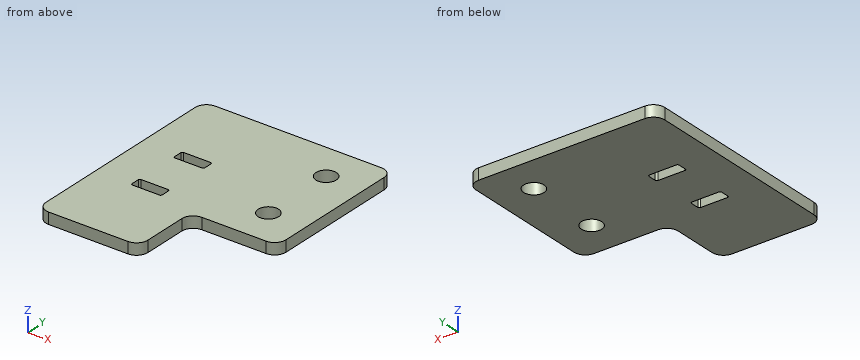
```python
from build123d import *

# Parameters (mm, degrees)
MODEL_R                         = 2.7
AUFSATZ_LINEAR_AUSTRAGEN1_DEPTH = 3


with BuildPart() as part:
    # Model → Aufsatz-Linear austragen1 (new body)
    with BuildSketch(Plane.XY):
        with BuildLine():
            Line((50, 20.75), (50, 54.75))
            ThreePointArc((50, 54.75), (49.121320344, 56.871320344), (47, 57.75))
            Line((47, 57.75), (3, 57.75))
            ThreePointArc((3, 57.75), (0.878679656, 56.871320344), (0, 54.75))
            Line((0, 54.75), (0, 3))
            ThreePointArc((0, 3), (0.878679656, 0.878679656), (3, 0))
            Line((3, 0), (24, 0))
            ThreePointArc((24, 0), (26.121320344, 0.878679656), (27, 3))
            Line((27, 3), (27, 14.75))
            ThreePointArc((27, 14.75), (27.878679656, 16.871320344), (30, 17.75))
            Line((30, 17.75), (47, 17.75))
            ThreePointArc((47, 17.75), (49.121320344, 18.628679656), (50, 20.75))
        make_face()
        with Locations((40, 27.75)):
            Circle(MODEL_R, mode=Mode.SUBTRACT)
        with Locations((40, 47.75)):
            Circle(MODEL_R, mode=Mode.SUBTRACT)
        with BuildLine():
            Line((17.1, 34.75), (9.9, 34.75))
            ThreePointArc((9.9, 34.75), (9.617157288, 34.867157288), (9.5, 35.15))
            Line((9.5, 35.15), (9.5, 37.35))
            ThreePointArc((9.5, 37.35), (9.617157288, 37.632842712), (9.9, 37.75))
            Line((9.9, 37.75), (17.1, 37.75))
            ThreePointArc((17.1, 37.75), (17.382842712, 37.632842712), (17.5, 37.35))
            Line((17.5, 37.35), (17.5, 35.15))
            ThreePointArc((17.5, 35.15), (17.382842712, 34.867157288), (17.1, 34.75))
        make_face(mode=Mode.SUBTRACT)
        with BuildLine():
            Line((17.100000028, 20.000000104), (9.900000028, 20.000000104))
            ThreePointArc((9.900000028, 20.000000104), (9.617157315, 20.117157391), (9.500000028, 20.400000104))
            Line((9.500000028, 20.400000104), (9.500000028, 22.600000104))
            ThreePointArc((9.500000028, 22.600000104), (9.617157315, 22.882842816), (9.900000028, 23.000000104))
            Line((9.900000028, 23.000000104), (17.100000028, 23.000000104))
            ThreePointArc((17.100000028, 23.000000104), (17.38284274, 22.882842816), (17.500000028, 22.600000104))
            Line((17.500000028, 22.600000104), (17.500000028, 20.400000104))
            ThreePointArc((17.500000028, 20.400000104), (17.38284274, 20.117157391), (17.100000028, 20.000000104))
        make_face(mode=Mode.SUBTRACT)
    extrude(amount=AUFSATZ_LINEAR_AUSTRAGEN1_DEPTH)


solid = part.part
```
CAD build for the part. Positions are in the model's coordinates, mm. Round coordinates to 2 decimals unless told otherwise and drop trailing zeros. Order: outer loops, then holes, each group sorted by start corner. A loop starts at its lowest first (then second) coordinate and runs counter-clockwise, first axis right, second up. Notation, with made-up numbers: (16.25, 11.5) - (52.25, 11.5) arc R12 cw to (52.25, 34.5) - close; hole circle Ø6 at (-10, 35). An arc over 180 degrees is marked (long way). Use CSV: the item, a comma, the result in double quotes. Start each with the question number.
1) Saw through at D-D (x = 33). List the corners of the cut face in (y, z), and give its area (3 significant figures).
2) Saw through at C-C (z = 1.5). Count the separate pieces of the cut face and the enclosed holes in it, and give its area (3 significant figures).
3) Saw through at A-A (x = 40). List the corners of the cut face in (y, z), and give its area (3 significant figures).
4) Pin check, flat tip, straight feed: pin 1 Ø6 at (x, y) = (17, 9) entering from -Z. Stop position of the tip, or through.
5) Saw through at B-B (y = 47.75). List the corners of the cut face in (x, z), and give its area (3 significant figures).
6) Wall check: L1, parallel to Y at x = 40, z = 2; L2, parallel to Y at x = 16.5, z = 0.7; L3, parallel to X at y = 22, z = 2.65. Give the ranges that are in metal, low to high. Write a range as [from, to].
Values follow:
1,outline,"(17.75, 0) - (57.75, 0) - (57.75, 3) - (17.75, 3) - close"
1,area,"120 mm2"
2,separate pieces,"1"
2,enclosed holes,"4"
2,area,"2,380 mm2"
3,outline,"(17.75, 0) - (25.05, 0) - (25.05, 3) - (17.75, 3) - close; (30.45, 0) - (45.05, 0) - (45.05, 3) - (30.45, 3) - close; (50.45, 0) - (57.75, 0) - (57.75, 3) - (50.45, 3) - close"
3,area,"87.6 mm2"
4,pin 1,"stops at z = 0"
5,outline,"(0, 0) - (37.3, 0) - (37.3, 3) - (0, 3) - close; (42.7, 0) - (50, 0) - (50, 3) - (42.7, 3) - close"
5,area,"134 mm2"
6,L1,"y = [17.75, 25.05], [30.45, 45.05], [50.45, 57.75]"
6,L2,"y = [0, 20], [23, 34.75], [37.75, 57.75]"
6,L3,"x = [0, 9.5], [17.5, 50]"
